Could you check a few things on this drawing? It's one solid part, dimensions in mm from its lowest x, y, z. Coordinates: 2 decimals unless noted, no trailing zeros. Order: outer loops, then holes, each group sorted by start corner. A loop starts at its lowest first (then second) coordinate and runs counter-clockwise, first axis right, second up. Notation, with made-up numbers: (-38, 81) - (0, 81) arc R12 ccw to (0, 85) - close; hole circle Ø11 at (-17, -20.5). An arc over 180 degrees is marked (long way). Answer in a Markdown table with one row per item. Add a question column.
Item 1: I want a section at D-D (x = 66). Please give me the cut outline in (y, z), plus the area to 3 significant figures.
Item 2: I want a section at C-C (z = 49.5). Please give me the cut outline in (x, y).
Item 3: I want a section at A-A (z = 66). Please give me the cut outline in (x, y).
Item 4: I want a section at B-B (x = 75). Please give me the cut outline in (y, z).
Item 5: If I drill on line 1 along X through (y, z) = (7.75, 66); line 2 along Z through (x, y) = (66.5, 7.75); line 3 along X through (y, z) = (9.25, 57), over which ranges is the centre line in solid material (lowest first)? Write a range as from..to.
Item 6: Will these pins go through, and if not, where does the flat tip stop? pin 1 Ø1.6 at (x, y) = (31.5, 9) entering from -Z; pin 2 Ø1.8 at (x, z) = (65, 66.5) entering from +Y; pin 3 Ø4.5 at (x, y) = (42.5, 9) entering from +Z.
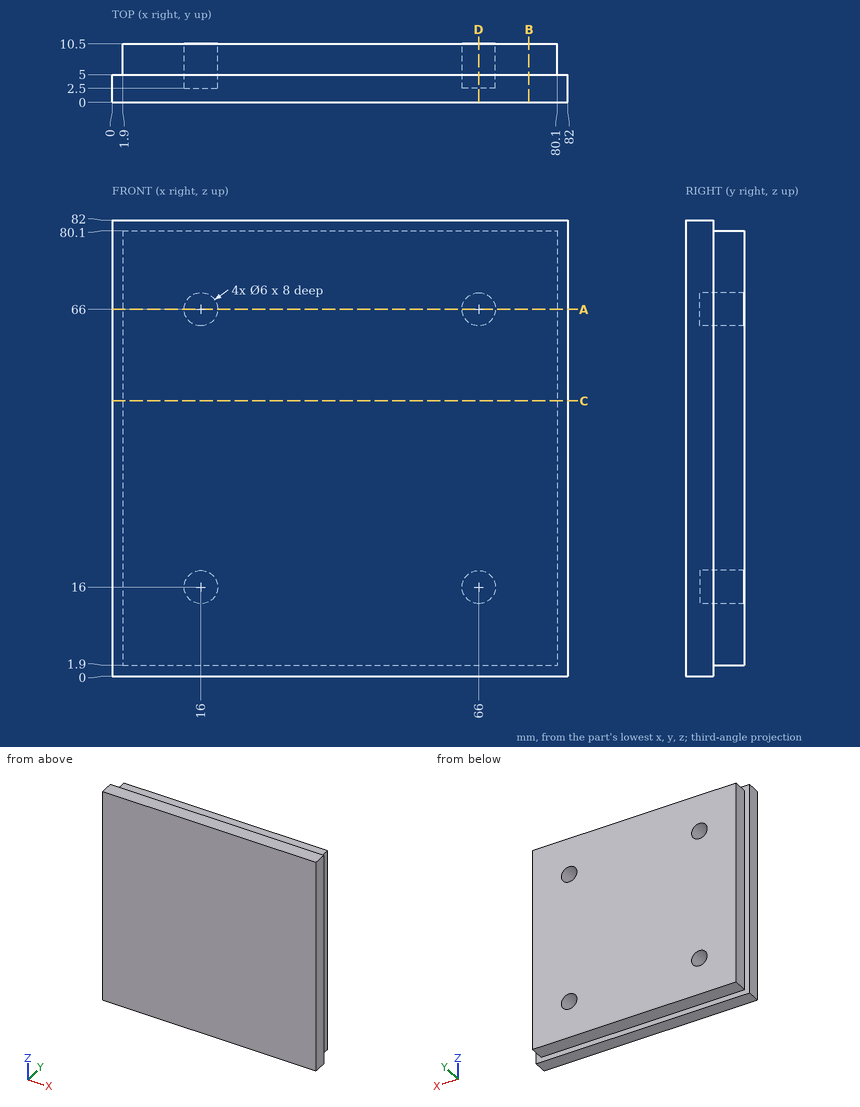
Values follow:
| question | item | result |
|---|---|---|
| 1 | outline | (0, 0) - (5, 0) - (5, 1.9) - (10.5, 1.9) - (10.5, 13) - (2.5, 13) - (2.5, 19) - (10.5, 19) - (10.5, 63) - (2.5, 63) - (2.5, 69) - (10.5, 69) - (10.5, 80.1) - (5, 80.1) - (5, 82) - (0, 82) - close |
| 1 | area | 744 mm^2 |
| 2 | outline | (0, 0) - (82, 0) - (82, 5) - (80.1, 5) - (80.1, 10.5) - (1.9, 10.5) - (1.9, 5) - (0, 5) - close |
| 3 | outline | (0, 0) - (82, 0) - (82, 5) - (80.1, 5) - (80.1, 10.5) - (69, 10.5) - (69, 2.5) - (63, 2.5) - (63, 10.5) - (19, 10.5) - (19, 2.5) - (13, 2.5) - (13, 10.5) - (1.9, 10.5) - (1.9, 5) - (0, 5) - close |
| 4 | outline | (0, 0) - (5, 0) - (5, 1.9) - (10.5, 1.9) - (10.5, 80.1) - (5, 80.1) - (5, 82) - (0, 82) - close |
| 5 | line 1 | x = 1.9..13, 19..63, 69..80.1 |
| 5 | line 2 | z = 1.9..13.04, 18.96..63.04, 68.96..80.1 |
| 5 | line 3 | x = 1.9..80.1 |
| 6 | pin 1 | stops at z = 1.9 |
| 6 | pin 2 | stops at y = 2.5 |
| 6 | pin 3 | stops at z = 80.1 |
